For this review, take the finished solid that the model builds, in its own axes (mm). A direction names the side the tool comes from. Coordinates: 2 decimals unless noted, no trailing zeros. Loops run counter-clockwise (first coordinate to the right, second up) from the corner with the lowest first, then second, coordinate; pieces in that order, holes last.
Autodesk Inventor part; units mm, degrees
ref_plane "YZ Plane" through (0, 0, 0) normal (1, 0, 0) x (0, 1, 0)
ref_plane "XZ Plane" through (0, 0, 0) normal (0, 1, 0) x (-1, 0, 0)
ref_plane "XY Plane" through (0, 0, 0) normal (0, 0, 1) x (1, 0, 0)
sketch "Sketch1" plane through (0, 0, 0) normal (0, 0, 1) x (1, 0, 0)
  line L0 (0, 0) -> (41, 0)
  line L1 (41, 0) -> (41, 55.5)
  line L2 (41, 55.5) -> (0, 55.5)
  line L3 (0, 55.5) -> (0, 0)
  dimension "d0" = 41
  dimension "d1" = 55.5
extrude "Extrusion1" add sketch "Sketch1" along normal blind 3
sketch "Sketch2" plane through (0, 0, 3) normal (0, 0, 1) x (1, 0, 0)
  line L0 (0, 0) -> (41, 0)
  line L1 (0, 55.5) -> (0, 0)
  line L2 (41, 0) -> (41, 55.5)
  line L3 (41, 55.5) -> (0, 55.5)
  line L4 (0, 0) -> (10, 0)
  line L5 (10, 0) -> (10, 3)
  line L6 (10, 3) -> (0, 3)
  line L7 (0, 3) -> (0, 0)
  line L8 (41, 0) -> (31, 0)
  line L9 (31, 0) -> (31, 3)
  line L10 (31, 3) -> (41, 3)
  line L11 (41, 3) -> (41, 0)
  line L12 (15.5, 52.5) -> (25.5, 52.5)
  line L13 (25.5, 52.5) -> (25.5, 55.5)
  line L14 (25.5, 55.5) -> (15.5, 55.5)
  line L15 (15.5, 55.5) -> (15.5, 52.5)
  line L16 (15.5, 52.5) -> (25.5, 55.5) construction
  line L17 (25.5, 52.5) -> (15.5, 55.5) construction
  line L18 (15.5, 52.5) -> (25.5, 52.5) construction
  line L19 (10, 0) -> (31, 0)
  line L20 (31, 0) -> (31, 3)
  line L21 (31, 3) -> (10, 3)
  line L22 (10, 3) -> (10, 0)
  point P0 (20.5, 54)
  point P1 (20.5, 52.5)
  dimension "d35" = 10
  dimension "d36" = 3
  dimension "d37" = 10
  dimension "d38" = 3
  dimension "d39" = 10
  dimension "d40" = 0
  dimension "d41" = 3
  dimension "d44" = 41
  dimension "d45" = 20.5
sketch "Sketch3" plane through (0, 0, 3) normal (0, 0, 1) x (1, 0, 0)
  line L0 (41, 0) -> (41, 55.5)
  line L1 (41, 55.5) -> (38, 55.5)
  line L2 (38, 55.5) -> (38, 40.5)
  line L3 (38, 40.5) -> (41, 40.5)
  line L4 (41, 40.5) -> (41, 55.5)
  point P0 (0, 0)
  dimension "d16" = 3
  dimension "d17" = 15
extrude "Extrusion3" cut sketch "Sketch3" against normal through all
sketch "Sketch4" plane through (0, 0, 3) normal (0, 0, 1) x (1, 0, 0)
  line L0 (38, 55.5) -> (0, 55.5)
  line L1 (41, 0) -> (41, 40.5)
  line L2 (41, 20) -> (51, 20)
  line L3 (51, 20) -> (51, 55.5)
  line L4 (51, 55.5) -> (41, 55.5)
  line L5 (41, 55.5) -> (41, 20)
  line L6 (0, 0) -> (41, 0)
  point P0 (69, 46)
  point P1 (89, 0)
  point P2 (0, 55.5)
  dimension "d20" = 10
  dimension "d21" = 20
extrude "Extrusion4" add sketch "Sketch4" against normal blind 3
sketch "Sketch5" plane through (0, 0, 3) normal (0, 0, 1) x (1, 0, 0)
  line L0 (0, 55.5) -> (0, 0)
  line L1 (0, 55.5) -> (-10, 55.5)
  line L2 (-10, 55.5) -> (-10, 20)
  line L3 (-10, 20) -> (0, 20)
  line L4 (0, 20) -> (0, 55.5)
  line L5 (0, 0) -> (41, 0)
  point P0 (20, 0)
  dimension "d24" = 10
  dimension "d25" = 20
extrude "Extrusion5" add sketch "Sketch5" against normal blind 3
sketch "Sketch6" plane through (0, 0, 3) normal (0, 0, 1) x (1, 0, 0)
  point P0 (0, 0)
sketch "Sketch7" plane through (0, 0, 3) normal (0, 0, 1) x (1, 0, 0)
  line L0 (38, 55.5) -> (-10, 55.5)
  line L1 (0, 55.5) -> (3, 55.5)
  line L2 (3, 55.5) -> (3, 40.5)
  line L3 (3, 40.5) -> (0, 40.5)
  line L4 (0, 40.5) -> (0, 55.5)
  point P0 (0, 0)
  point P1 (30, 46)
  point P2 (-10, 55.5)
  dimension "d28" = 3
  dimension "d29" = 15
extrude "Extrusion6" cut sketch "Sketch7" against normal through all
fillet "Fillet1" radius 2 10 edges at (0, 55.5, 1.5) (3, 55.5, 1.5) (-10, 55.5, 1.5) (38, 55.5, 1.5) (41, 55.5, 1.5) (51, 55.5, 1.5) (51, 20, 1.5) (41, 20, 1.5) (-10, 20, 1.5) (0, 20, 1.5)
extrude "Extrusion7" cut sketch "Sketch2" against normal through all contours L5 L21 L9 L0 | L3 L13 L12 L15
properties part number "front_left_v2"
Q1. Consider section C-C (x = 29.5). State the section outline as (y, z) points.
Q2. For pin 1 Ø12 at (x, y) = (29.5, 46) entering from -Z; pin 2 Ø1.5 at (x, z) = (40, 1) entering from +Y; pin 3 Ø1.5 at (x, z) = (23, 2) entering from +Y; pin 4 Ø1.5 at (y, z) = (1.5, 1) entering from +X, all flat-tipped, find the tip position at first contact; note any pin that passes through.
Q3. Wall thickness on probe 1 along X at (y, z) = (50.5, 0.9); probe 2 along Y at (x, z) = (48.5, 0.6); probe 3 along Y at (x, z) = (19, 1.3): over which ranges is each line inside the solid? List them lowest first.
Q4. The part is to be moulded in two halves that separate along X. For faces 1 (the face through (25.5, 54, 2)), 2 (the face through (-9.43, 54.9, 1.48)), 3 (the face through (46, 20, 2)), 4 (the face through (3, 47, 2)), say which applies: +X half, -X half, draft (parallel to the pull), parting line (faces both ways), or undercut.
Q5. Consider section B-B (y = 7). State the section outline as (x, z) points, then the cut area to 3 significant figures.
Q6. Machinability: for faces 5 (the face through (3.57, 54.9, 1.48)), 6 (the face through (0, 9, 1)), 7 (the face through (41, 9, 1)), 8 (the face through (10, 1, 2)), which of the approach directions +Z, -Z, +X, -X, +Y, -Y give a long, thin tool a straight path to every point of the face, cutting with its end or side? Answer none if there is none.
Model answer:
1. outline: (3, 0) - (55.5, 0) - (55.5, 3) - (3, 3) - close
2. pin 1: stops at z = 0
2. pin 2: stops at y = 40.5
2. pin 3: stops at y = 52.5
2. pin 4: stops at x = 41
3. probe 1: x = -10 to 0, 3 to 38, 41 to 51
3. probe 2: y = 20 to 55.5
3. probe 3: y = 3 to 52.5
4. face 1: undercut
4. face 2: -X half
4. face 3: draft
4. face 4: undercut
5. outline: (0, 0) - (41, 0) - (41, 3) - (0, 3) - close
5. area: 123 mm2
6. face 5: +Z, -Z, +Y
6. face 6: +Z, -Z, -X, -Y
6. face 7: +Z, -Z, +X, -Y
6. face 8: +Z, -Z, -Y
